Check sheet for the modelled part. Datum: model origin and axes. Units: mm. A direction names the side the tool comes from. Give positions to 0.01 mm unless a question says otherwise; leave off trailing zeros. Order: outer loops, then holes, each group sorted by start corner. A loop starts at its lowest first (then second) coordinate and runs counter-clockwise, first axis right, second up. Notation, with made-up numbers: (-32, 22.25) -> (-1, 22.25) arc R17 cw to (-1, 49.25) -> close; hole circle Ø10 at (-26.5, 7). An arc over 180 degrees is marked (long way). One line per question, with ' | ' between items.
```python
from build123d import *

# Parameters (mm, degrees)
F0_R     = 8
F1_DEPTH = 14
F2_W     = 0.63
F2_H     = 0.63
F3_DEPTH = 7
F6_W     = 0.685
F6_H     = 0.63
F6_W_2   = 0.63
F7_DEPTH = 7


with BuildPart() as f1:
    # F0 (on Right) → F1 (new body)
    with BuildSketch(Plane.YZ):
        Circle(F0_R)
    extrude(amount=F1_DEPTH)

    # F2 (on Right) → F3 (cut)
    with BuildSketch(Plane.YZ):
        Rectangle(F2_W, F2_H)
    extrude(amount=F3_DEPTH, mode=Mode.SUBTRACT)

    # F6 (on offset) → F7 (cut)
    with BuildSketch(Plane(origin=(7, 0, 0), x_dir=(0, 1, 0), z_dir=(-1, 0, 0))):
        with Locations((-0.6575, 0)):
            Rectangle(F6_W, F6_H)
        Rectangle(F6_W_2, F6_H)
        with Locations((0.6575, 0)):
            Rectangle(F6_W, F6_H)
    extrude(amount=F7_DEPTH, mode=Mode.SUBTRACT)


solid = f1.part
```
Q1. Section check D-D (z = 2.5). Enter the section's corners in (x, y).
Result sheet:
outline: (0, -7.6) -> (14, -7.6) -> (14, 7.6) -> (0, 7.6) -> close
Q2. Thickness scan on line 1 (Z direction, x = 0.5, y = 0.75) (3 decimals); line 2 (Z direction, x = 11, y = -0.25); line 3 (Z direction, x = 7.25, y = -5) (3 decimals). Record the ranges inside material, lowest first.
Result sheet:
line 1: z = -7.965 to -0.315, 0.315 to 7.965 | line 2: z = -8 to 8 | line 3: z = -6.245 to 6.245
Q3. Section check A-A (x = 3.25). Enter the section's corners in (y, z) (3 decimals).
Result sheet:
outline: circle Ø16 at (0, 0); hole (-1, -0.315) -> (1, -0.315) -> (1, 0.315) -> (-1, 0.315) -> close
Q4. Depth check by flat-ended pin: pin 1 Ø0.6 at (x, y) = (5, 0.5) entering from -Z; pin 2 Ø1.5 at (x, y) = (11.5, -3) entering from +Z; pin 3 Ø1 at (x, y) = (7.5, 1.5) entering from +Z. Enter the tip coordinate at first touch or a pass-through.
Result sheet:
pin 1: stops at z = -8 | pin 2: stops at z = 7.68 | pin 3: stops at z = 7.94
Q5. Mould release check, pull along Y, two halves, no side actions. Record for faces 3 (the face through (14, 0, 0)), 4 (the face through (6.9, -1.73, -7.81)), 5 (the face through (4, 0, 0.315)): pulls with the +Y half, pulls with the -Y half, needs draft (parallel to the pull), parting line crosses it, or undercut.
Result sheet:
face 3: needs draft | face 4: parting line crosses it | face 5: undercut
Q6. Section check B-B (y = 0). Enter the section's corners in (x, z) (3 decimals), and give its area (3 significant figures).
Result sheet:
outline: (0, -8) -> (14, -8) -> (14, 8) -> (0, 8) -> (0, 0.315) -> (7, 0.315) -> (7, -0.315) -> (0, -0.315) -> close | area: 220 mm2
Q7. Access from +Z, -Z, +X, -X, +Y, -Y to the whole of each face (thin tool, end or side, straight path). Record for faces 1 (the face through (3, 0, -0.315)), 2 (the face through (0, 2, 0)).
Result sheet:
face 1: -X | face 2: +Z, -Z, -X, +Y, -Y
Q8. Section check C-C (x = 7.5). Enter the section's corners in (y, z).
Result sheet:
outline: circle Ø16 at (0, 0)
